Geometry check sheet. Reference: the model listing, model coordinates, mm. A direction names the side the tool comes from. Coordinates: 2 decimals unless noted, no trailing zeros. Write each loop counter-clockwise with the first axis right and the second up, starting at its lowest first coordinate (ties: lowest second). Pieces come first, ordered by that corner, then holes. Notation, with made-up numbers: (44, -23.5) -> (89, -23.5) arc R34 cw to (89, 11.5) -> close; hole circle Ø7 at (-31, 51). An arc over 180 degrees is marked (long way). Answer in a Markdown table with one row per item. Add a question column.
1. Cross-section at B-B on x = 8.5. Record the cut outline in (y, z), and give its area (3 significant figures).
2. Scan lines: L1, parallel to Y at x = 25, z = 10.5; L2, parallel to X at y = 11, z = 3; L3, parallel to X at y = 2, z = 7.25. Record each from-to range of solid material in increasing order. Write a range as from..to.
3. Cross-section at D-D on z = 8. Give the number of separate pieces and of enclosed holes in the cut face, and give its area (3 significant figures).
4. Cross-section at A-A on y = 13. Record the cut outline in (x, z) (1 decimal), and give its area (3 significant figures).
5. Cross-section at C-C on z = 3.5. Record the cut outline in (x, y).
6. Depth check by flat-ended pin: P1, Ø3, axis at x = 29, z = 4.5, coming from the +Y side; P2, Ø7, axis at x = 22, z = 6, coming from the +Y side; P3, Ø4, axis at x = 5.5, y = 17.5, coming from the +Z side. Enter the tip coordinate at first touch or a pass-through.
7. Mould release check, pull along Z, two halves, no side actions. Record for faces 1 (the flat face through (17, 25, 7)), 2 (the cylindrical face through (32, 26.5, 11.4)), 3 (the flat face through (23.15, 1.52, 8.43)), 4 (the flat face through (10.85, 1.52, 8.43)): pulls with the +Z half, pulls with the -Z half, needs draft (parallel to the pull), parting line crosses it, or undercut.
8. Set-up check for faces 5 (the flat face through (31.5, 14, 2)), 6 (the cylindrical face through (2, 26.5, 11.4)), 7 (the flat face through (29.01, 1.52, 9.36)): record each of +Z, -Z, +X, -X, +Y, -Y from which the full face is reachable in a straight line by a thin tool's end or side.
Autodesk Fusion 360 part; units mm, degrees
sketch "Skizze1" plane through (0, 0, 0) normal (0, 1, 0) x (1, 0, 0)
  line L0 (0, 0) -> (0, -13.5)
  line L1 (0, -13.5) -> (34, -13.5)
  line L2 (34, -13.5) -> (34, 0)
  line L3 (34, 0) -> (0, 0)
  dimension "d1" = 13.5
  dimension "d2" = 34
extrude "Extrusion1" add sketch "Skizze1" along normal blind 3
sketch "Skizze2" plane through (0, 3, 0) normal (0, 1, 0) x (-1, 0, 0)
  line L0 (-34, 0) -> (0, 0)
  line L1 (0, 0) -> (0, 13.5)
  line L2 (0, 13.5) -> (-34, 13.5)
  line L3 (-34, 13.5) -> (-34, 0)
  line L4 (-34, 0) -> (-31.5, 0)
  line L5 (-31.5, 0) -> (-31.5, 5)
  line L6 (-31.5, 5) -> (-29.5, 5)
  line L7 (-29.5, 5) -> (-29.5, 0)
  line L8 (0, 0) -> (-2.5, 0)
  line L9 (-2.5, 0) -> (-2.5, 5)
  line L10 (-2.5, 5) -> (-4.5, 5)
  line L11 (-4.5, 5) -> (-4.5, 0)
  line L12 (-4.5, 5) -> (-4.5, 13.5)
  line L13 (-29.5, 5) -> (-29.5, 13.5)
  line L14 (-4.5, 0) -> (-29.5, 0)
  line L15 (-4.5, 0) -> (-17, 13.5)
  line L16 (-29.5, 0) -> (-17, 13.5)
  line L17 (-25.3803, 4.4492) -> (-29.5, 0)
  line L18 (-31.5, 5) -> (-31.5, 13.5)
  line L19 (-17, 0) -> (-17, 13.5)
  line L20 (-29.5, 0) -> (-26.7824, 2.935)
  line L21 (-26.7824, 2.935) -> (-23.8473, 0.2174)
  line L22 (-26.7824, 2.935) -> (-31.1849, 7.0115)
  line L23 (-31.1849, 7.0115) -> (-26.7688, 11.7809)
  line L24 (-26.7688, 11.7809) -> (-19.4312, 4.9869)
  line L25 (-19.4312, 4.9869) -> (-23.8473, 0.2174)
  line L26 (-4.5, 0) -> (-7.2176, 2.935)
  line L27 (-7.2176, 2.935) -> (-10.1527, 0.2174)
  line L28 (-10.1527, 0.2174) -> (-7.2176, 2.935)
  line L29 (-7.2176, 2.935) -> (-2.8151, 7.0115)
  line L30 (-2.8151, 7.0115) -> (-7.2312, 11.7809)
  line L31 (-7.2312, 11.7809) -> (-14.5688, 4.9869)
  line L32 (-14.5688, 4.9869) -> (-10.1527, 0.2174)
  line L33 (-29.5, 0) -> (-29.5, 5)
  line L34 (-31.5, 5) -> (-29.5, 5)
  line L35 (-19.4312, 4.9869) -> (-19.4286, 0)
  line L36 (-14.5688, 4.9869) -> (-14.5319, 0)
  line L37 (-2.8151, 7.0115) -> (-2.5, 5)
  line L38 (-31.1849, 7.0115) -> (-31.5, 5)
  dimension "d5" = 2.5
  dimension "d6" = 2
  dimension "d7" = 2.5
  dimension "d8" = 5
  dimension "d9" = 2
  dimension "d10" = 4
  dimension "d11" = 4
  dimension "d12" = 6
  dimension "d13" = 6.5
  dimension "d14" = 10
  dimension "d15" = 4
  dimension "d16" = 4
  dimension "d17" = 6
  dimension "d18" = 6.5
  dimension "d19" = 10
extrude "Extrusion2" cut sketch "Skizze2" against normal blind 10 contours L13 L16 L17 L22 L23 L24 | L16 L17 L21 L24 L25 | L13 L22 L23 | L12 L15 L29 L30 L31 | L15 L27 L28 L31 L32 | L12 L29 L30
extrude "Extrusion3" add sketch "Skizze2" along normal blind 21 contours L0 L5 L6 L7 L33 L34 | L0 L14 L16 L17 L20 L21 L25 L35 | L7 L13 L16 L17 L20 L22 L33 | L6 L13 L22 L34 L38 | L0 L14 L15 L26 L27 L28 L32 L36 | L0 L9 L10 L11 | L11 L12 L15 L26 L29 | L10 L12 L29 L37
extrude "Extrusion4" add 2 faces at (5.0509, 24, 1.7391) (28.9491, 24, 1.7391) along direction (0, 1, 0) blind 1
sketch "Skizze3" plane through (0, 0, 0) normal (0, 0, -1) x (-1, 0, 0)
  line L0 (-34, 0) -> (0, 0)
  line L1 (0, 0) -> (0, 3)
  line L2 (0, 3) -> (-2.5, 3)
  line L3 (-2.5, 3) -> (-2.5, 25)
  line L4 (-2.5, 25) -> (-14.5319, 25)
  line L5 (-14.5319, 25) -> (-14.5319, 3)
  line L6 (-14.5319, 3) -> (-19.4286, 3)
  line L7 (-19.4286, 3) -> (-19.4286, 25)
  line L8 (-19.4286, 25) -> (-31.5, 25)
  line L9 (-31.5, 25) -> (-31.5, 3)
  line L10 (-31.5, 3) -> (-34, 3)
  line L11 (-34, 3) -> (-34, 0)
  line L12 (-34, 3) -> (-34, 25)
  line L13 (-34, 25) -> (0, 25)
  line L14 (0, 25) -> (0, 28)
  line L15 (0, 28) -> (-34, 28)
  line L16 (-34, 28) -> (-34, 25)
  line L17 (-17, 28) -> (-17, 21.0656)
  circle A0 centre (-17, 28) radius 6.9344
extrude "Extrusion5" add sketch "Skizze3" against normal blind 13.5 contours L8 L13 L15 L16 A0 | L4 L13 L14 L15 A0 | L8 L13 L15 L17 A0 | L15 A0 | L4 L13 L15 L17 A0
fillet "Abrundung1" radius 6 1 edges at (17, 34.9344, 13.5)
fillet "Abrundung2" radius 4 1 edges at (0, 26.5, 13.5)
fillet "Abrundung3" radius 4 1 edges at (34, 26.5, 13.5)
delete_face "Fläche löschen1" 1 faces at (33.9819, 26, 9.8802)
delete_face "Fläche löschen2" 1 faces at (0.0181, 26, 9.8802)
fillet "Abrundung4" radius 7 1 edges at (34, 26.5, 13.5)
fillet "Abrundung5" radius 7 1 edges at (0, 26.5, 13.5)
Results found:
| question | item | result |
|---|---|---|
| 1 | outline | (0, 0) -> (28, 0) -> (28, 13.5) -> (25, 13.5) -> (25, 1.75) -> (0, 1.75) -> close; (0, 10.61) -> (3, 10.61) -> (3, 13.5) -> (0, 13.5) -> close |
| 1 | area | 92.9 mm^2 |
| 2 | L1 | y = 0..3, 25..28 |
| 2 | L2 | x = 2.5..7.15, 12.73..14.55, 19.43..21.27, 26.85..31.5 |
| 2 | L3 | x = 0..3.04, 12.12..21.88, 30.96..34 |
| 3 | separate pieces | 4 |
| 3 | enclosed holes | 0 |
| 3 | area | 233 mm^2 |
| 4 | outline | (2.5, 0) -> (14.5, 0) -> (14.6, 5) -> (10.2, 0.2) -> (7.2, 2.9) -> (2.8, 7) -> (2.5, 5) -> close; (19.4, 0) -> (31.5, 0) -> (31.5, 5) -> (31.2, 7) -> (26.8, 2.9) -> (23.8, 0.2) -> (19.4, 5) -> close |
| 4 | area | 79.7 mm^2 |
| 5 | outline | (0, 0) -> (6.61, 0) -> (6.61, 25) -> (13.19, 25) -> (13.19, 0) -> (20.81, 0) -> (20.81, 25) -> (27.39, 25) -> (27.39, 0) -> (34, 0) -> (34, 3) -> (31.5, 3) -> (31.5, 25) -> (34, 25) -> (34, 28) -> (23.93, 28) arc R6.93 ccw to (10.07, 28) -> (0, 28) -> (0, 25) -> (2.5, 25) -> (2.5, 3) -> (0, 3) -> close; hole (14.56, 3) -> (19.43, 3) -> (19.43, 25) -> (14.56, 25) -> close |
| 6 | P1 | stops at y = 28 |
| 6 | P2 | stops at y = 34.77 |
| 6 | P3 | stops at z = 6.38 |
| 7 | face 1 | needs draft |
| 7 | face 2 | pulls with the +Z half |
| 7 | face 3 | undercut |
| 7 | face 4 | undercut |
| 8 | face 5 | +Z, -Z, +X |
| 8 | face 6 | +Z, -X, +Y |
| 8 | face 7 | -Y |
